from build123d import *

# Parameters (mm, degrees)
BOSS_EXTRUDE1_DEPTH = 3.571875
SHELL1_T            = -0.6096
EXTRUDE_THIN3_DEPTH = 3.571875
EXTRUDE_THIN4_DEPTH = 3.571875
EXTRUDE_THIN6_DEPTH = 1.190625
FILLET4_R           = 0.4572
FILLET5_R           = 0.2286
FILLET6_R           = 0.1143
FILLET7_R           = 0.508


with BuildPart() as part:
    # Sketch1 → Boss-Extrude1 (new, symmetric)
    with BuildSketch(Plane.XY):
        Polygon((-5.6096, 33.514075028), (-5.6096, 37.873675028), (5.6096, 37.873675028), (5.6096, 33.514075028), (5, 33.514075028), (-5, 33.514075028), align=None)
    extrude(amount=BOSS_EXTRUDE1_DEPTH, both=True)

    # Shell1
    shell1_openings = [part.faces().sort_by_distance(p)[0] for p in [
        (0, 35.693875028, 3.571875),
        (0, 33.514075028, 0),
        (0, 35.693875028, -3.571875),
    ]]
    offset(amount=SHELL1_T, openings=shell1_openings, kind=Kind.INTERSECTION)

    # Sketch5 → Extrude-Thin3 (add, symmetric)
    with BuildSketch(Plane.XY):
        with BuildLine():
            ThreePointArc((5, 33.514075028), (11.90262143, 31.725712413), (18.278169619, 28.532468179))
            Line((18.278169619, 28.532468179), (18.606998664, 29.045774734))
            ThreePointArc((18.606998664, 29.045774734), (12.116752698, 32.296466265), (5.089951306, 34.117001991))
            Line((5.089951306, 34.117001991), (5, 33.514075028))
        make_face()
    extrude(amount=EXTRUDE_THIN3_DEPTH, both=True)

    # Sketch6 → Extrude-Thin4 (add, symmetric)
    with BuildSketch(Plane.XY):
        with BuildLine():
            ThreePointArc((-5, 33.514075028), (-11.439087927, 31.895775463), (-17.43901324, 29.052952384))
            ThreePointArc((-17.43901324, 29.052952384), (-17.647474534, 28.911954573), (-17.839493718, 28.749273517))
            Line((-17.839493718, 28.749273517), (-20.819129436, 25.934444001))
            ThreePointArc((-20.819129436, 25.934444001), (-20.883929256, 25.875496119), (-20.950901421, 25.819028441))
            ThreePointArc((-20.950901421, 25.819028441), (-24.112077535, 22.894763964), (-26.868805255, 19.586469927))
            ThreePointArc((-26.868805255, 19.586469927), (17.263572049, -28.417100135), (-5, 32.871910501))
            Line((-5, 32.871910501), (-5.091669173, 33.474578671))
            ThreePointArc((-5.091669173, 33.474578671), (17.580079524, -28.938094548), (-27.361413486, 19.945565026))
            ThreePointArc((-27.361413486, 19.945565026), (-24.554144376, 23.314512779), (-21.335011782, 26.292390238))
            ThreePointArc((-21.335011782, 26.292390238), (-21.285580426, 26.334068357), (-21.237752451, 26.377577087))
            Line((-21.237752451, 26.377577087), (-18.258116733, 29.192406602))
            ThreePointArc((-18.258116733, 29.192406602), (-18.015805435, 29.397695767), (-17.752745643, 29.575622585))
            ThreePointArc((-17.752745643, 29.575622585), (-11.644880107, 32.469588794), (-5.089951306, 34.117001991))
            Line((-5.089951306, 34.117001991), (-5, 33.514075028))
        make_face()
    extrude(amount=EXTRUDE_THIN4_DEPTH, both=True)

    # Sketch9 → Extrude-Thin6 (add, symmetric)
    with BuildSketch(Plane.XY):
        with BuildLine():
            ThreePointArc((-5, 32.871910501), (-11.269306607, 31.282027246), (-17.112208653, 28.508504258))
            Line((-17.112208653, 28.508504258), (-17.425941056, 29.031174459))
            ThreePointArc((-17.425941056, 29.031174459), (-11.47591621, 31.855546759), (-5.091669173, 33.474578671))
            Line((-5.091669173, 33.474578671), (-5, 32.871910501))
        make_face()
    extrude(amount=EXTRUDE_THIN6_DEPTH, both=True)

    # Fillet4
    fillet4_edges = [part.edges().sort_by_distance(p)[0] for p in [
        (-5.6096, 37.873675028, 0),
        (5.6096, 37.873675028, 0),
        (5, 33.514075028, 0),
        (-5, 33.514075028, 0),
    ]]
    fillet(fillet4_edges, radius=FILLET4_R)

    # Fillet5
    fillet5_edges = [part.edges().sort_by_distance(p)[0] for p in [
        (5.6096, 34.035420036, 0),
        (-5.6096, 34.035420036, 0),
    ]]
    fillet(fillet5_edges, radius=FILLET5_R)

    # Fillet6
    fillet6_edges = [part.edges().sort_by_distance(p)[0] for p in [
        (5, 37.264075028, 0),
        (-5, 37.264075028, 0),
    ]]
    fillet(fillet6_edges, radius=FILLET6_R)

    # Fillet7
    fillet7_edges = [part.edges().sort_by_distance(p)[0] for p in [
        (18.442584141, 28.789121456, -3.571875),
        (18.442584141, 28.789121456, 3.571875),
        (-5.045834586, 33.173244586, -3.571875),
        (-5.045834586, 33.173244586, 3.571875),
        (-17.269074855, 28.769839358, 1.190625),
        (-17.269074855, 28.769839358, -1.190625),
    ]]
    fillet(fillet7_edges, radius=FILLET7_R)


solid = part.part
Source: CAD feature listing. Evaluate the final solid. Frame: model axes, mm. A direction names the side the tool comes from. Round coordinates to 2 decimals unless told otherwise and drop trailing zeros. Loops run counter-clockwise (first coordinate to the right, second up) from the corner with the lowest first, then second, coordinate; pieces in that order, holes last.
Q1. Access query for faces 4 (the face through (5, 36, 0)), 5 (the face through (-5.61, 36, 0)), 6 (the face through (-11, 31.7, -1.191)), 7 (the face through (-11, 31.7, 1.191)). Directions: +Z, -Z, +X, -X, +Y, -Y. A direction counts if a zero-diameter tool reaches every point of the face in a straight line with its end or side. Return the directions, or none.
Q2. First-contact query: P1, Ø4, axis at y = 27.5, z = -1.5, coming from the -X side; P2, Ø3.5, axis at x = 2, z = 1, coming from the -Y side; P3, Ø3, axis at x = -15, z = -1.5, coming from the -Y side. Flat tips, straight axial feed; report the tip coordinate or a pass-through.
Q3. Section D-D, the plane x = 27. Return loops of the section in (y, z), plus the area to 3 significant figures.
Q4. Mould query, pull axis X, two halves, no side actions, for faces 1 (the face through (-19.31, 27.36, 0.05)), 2 (the face through (5.61, 36, 0)), 3 (the face through (-19.769, 27.765, 0.05)). Classes: pulls with the +X half, pulls with the -X half, needs draft (parallel to the pull), parting line crosses it, or undercut.
Q5. Section B-B, the plane x = 0. Return loops of the section in (y, z), plus the area to 3 significant figures.
Q6. Ray query, line 1 (Y direction, x = 0, z = -1.75); line 2 (X direction, y = 0, z = 1); line 3 (Y direction, x = -1, z = -1.5). Return the intervals inside material, ascending.
Q7. Section A-A, the plane y = 0. Return loops of the section in (x, z), plus the area to 3 significant figures.
Solutions:
1. face 4: +Z, -Z
1. face 5: +Z, -Z, -X, +Y
1. face 6: -Z
1. face 7: +Z
2. P1: stops at x = -22.28
2. P2: stops at y = -33.86
2. P3: stops at y = -31.05
3. outline: (-20.43, -3.57) - (-19.41, -3.57) - (-19.41, 3.57) - (-20.43, 3.57) - close; (19.41, -3.57) - (20.43, -3.57) - (20.43, 3.57) - (19.41, 3.57) - close
3. area: 14.7 mm2
4. face 1: undercut
4. face 2: pulls with the +X half
4. face 3: pulls with the -X half
5. outline: (-33.86, -3.57) - (-33.25, -3.57) - (-33.25, 3.57) - (-33.86, 3.57) - close; (33.25, -3.57) - (33.86, -3.57) - (33.86, 3.57) - (33.25, 3.57) - close; (37.26, -3.57) - (37.87, -3.57) - (37.87, 3.57) - (37.26, 3.57) - close
5. area: 13.1 mm2
6. line 1: y = -33.86 to -33.25, 33.25 to 33.86, 37.26 to 37.87
6. line 2: x = -33.86 to -33.25, 33.25 to 33.86
6. line 3: y = -33.84 to -33.23, 33.23 to 33.84, 37.26 to 37.87
7. outline: (-33.86, -3.57) - (-33.25, -3.57) - (-33.25, 3.57) - (-33.86, 3.57) - close; (33.25, -3.57) - (33.86, -3.57) - (33.86, 3.57) - (33.25, 3.57) - close
7. area: 8.71 mm2
